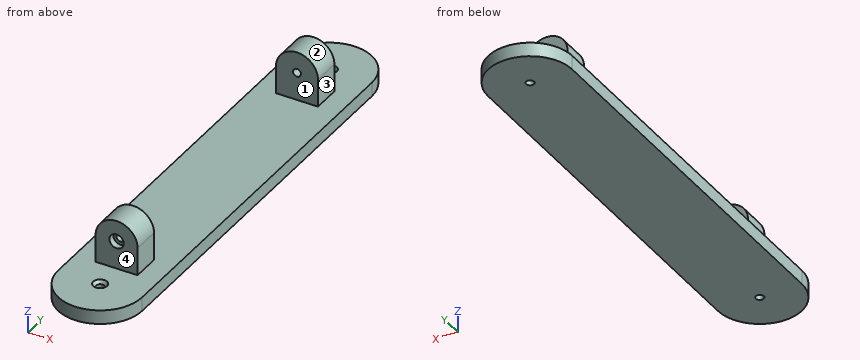
from build123d import *

# Parameters (mm, degrees)
BOSS_EXTRUDE1_DEPTH                             = 6.35
CSK_FOR_M3_FLAT_HEAD_MACHINE_SCREW1_D           = 3.6
CSK_FOR_M3_FLAT_HEAD_MACHINE_SCREW1_CSINK_D     = 6.3
CSK_FOR_M3_FLAT_HEAD_MACHINE_SCREW1_CSINK_ANGLE = 90
SKETCH3_W                                       = 19.05
SKETCH3_H                                       = 12.7
BOSS_EXTRUDE2_DEPTH                             = 12.7
BOSS_EXTRUDE5_DEPTH                             = 12.7
CBORE_FOR_M3_SHCS1_D                            = 3.6
CBORE_FOR_M3_SHCS1_CBORE_D                      = 6.5
CBORE_FOR_M3_SHCS1_CBORE_DEPTH                  = 3


with BuildPart() as part:
    # Sketch1 → Boss-Extrude1 (new body)
    with BuildSketch(Plane.XY):
        with BuildLine():
            Line((0, 0), (38.1, 0))
            Line((38.1, 0), (38.1, 88.9))
            ThreePointArc((38.1, 88.9), (19.05, 107.95), (0, 88.9))
            Line((0, 88.9), (0, 0))
        make_face()
    boss_extrude1 = extrude(amount=BOSS_EXTRUDE1_DEPTH)

    # CSK for M3 Flat Head Machine Screw1 (through all)
    with Locations(Plane(origin=(19.05, 88.9, 6.35), x_dir=(1, 0, 0), z_dir=(0, 0, 1))):
        with Locations((0, 0)):
            csk_for_m3_flat_head_machine_screw1 = CounterSinkHole(CSK_FOR_M3_FLAT_HEAD_MACHINE_SCREW1_D / 2, CSK_FOR_M3_FLAT_HEAD_MACHINE_SCREW1_CSINK_D / 2, counter_sink_angle=CSK_FOR_M3_FLAT_HEAD_MACHINE_SCREW1_CSINK_ANGLE)

    # Sketch3 → Boss-Extrude2 (add)
    with BuildSketch(Plane.XY.offset(6.35)):
        with Locations((19.05, 69.85)):
            Rectangle(SKETCH3_W, SKETCH3_H)
    boss_extrude2 = extrude(amount=BOSS_EXTRUDE2_DEPTH)

    # Sketch6 → Boss-Extrude5 (add)
    with BuildSketch(Plane(origin=(0, 76.2, 0), x_dir=(1, 0, 0), z_dir=(0, 1, 0))):
        with BuildLine():
            Line((9.525, -19.05), (28.575, -19.05))
            ThreePointArc((28.575, -19.05), (19.05, -28.575), (9.525, -19.05))
        make_face()
    boss_extrude5 = extrude(amount=-BOSS_EXTRUDE5_DEPTH)

    # CBORE for M3 SHCS1 (through all)
    with Locations(Plane(origin=(0, 76.2, 0), x_dir=(1, 0, 0), z_dir=(0, 1, 0))):
        with Locations((19.05, -19.05)):
            cbore_for_m3_shcs1 = CounterBoreHole(CBORE_FOR_M3_SHCS1_D / 2, CBORE_FOR_M3_SHCS1_CBORE_D / 2, CBORE_FOR_M3_SHCS1_CBORE_DEPTH)

    # Mirror1: Boss-Extrude1, CSK for M3 Flat Head Machine Screw1, Boss-Extrude2, Boss-Extrude5, CBORE for M3 SHCS1 across plane
    add(boss_extrude1.mirror(Plane.ZX))
    add(csk_for_m3_flat_head_machine_screw1.mirror(Plane.ZX), mode=Mode.SUBTRACT)
    add(boss_extrude2.mirror(Plane.ZX))
    add(boss_extrude5.mirror(Plane.ZX))
    add(cbore_for_m3_shcs1.mirror(Plane.ZX), mode=Mode.SUBTRACT)


solid = part.part
Work out the finished part from the listing and answer in its coordinate system (mm). Face numbers are marked on the shaded views. A direction names the side the tool comes from. Coordinates: 2 decimals unless noted, no trailing zeros. Write each loop counter-clockwise with the first axis right and the second up, starting at its lowest first coordinate (ties: lowest second). Pieces come first, ordered by that corner, then holes.
1. The part is cut by section C-C, the plane x = 13. Write down the section's boundary in (y, z), and give its area (3 significant figures).
Results list:
outline: (-106.96, 0) - (106.96, 0) - (106.96, 6.35) - (76.2, 6.35) - (76.2, 26.41) - (63.5, 26.41) - (63.5, 6.35) - (-63.5, 6.35) - (-63.5, 26.41) - (-76.2, 26.41) - (-76.2, 6.35) - (-106.96, 6.35) - close
area: 1,870 mm2
2. The part is cut by section D-D, the plane z = 25.75. Write down the section's boundary in (x, y).
Results list:
outline: (12.28, -76.2) - (25.82, -76.2) - (25.82, -63.5) - (12.28, -63.5) - close; (12.28, 63.5) - (25.82, 63.5) - (25.82, 76.2) - (12.28, 76.2) - close
3. The part is cut by section B-B, the plane z = 12.5. Write down the section's boundary in (x, y) (3 decimals), and give its area (3 significant figures).
Results list:
outline: (9.525, -76.2) - (28.575, -76.2) - (28.575, -63.5) - (9.525, -63.5) - close; (9.525, 63.5) - (28.575, 63.5) - (28.575, 76.2) - (9.525, 76.2) - close
area: 484 mm2
4. For the marked faces 1, 2, 3 and 4, determine the directions among +Z, -Z, +X, -X, +Y, -Y from which every point of the face is accessible in a straight line to the end or side of a thin tool.
Results list:
face 1: +Z, +X, -X
face 2: +Z, +Y, -Y
face 3: +Z, +X, +Y, -Y
face 4: +Z, +X, -X, -Y
5. The part is cut by section A-A, the plane y = 70. Write down the section's boundary in (x, z) (3 decimals), and give its area (3 significant figures).
Results list:
outline: (0, 0) - (38.1, 0) - (38.1, 6.35) - (28.575, 6.35) - (28.575, 19.05) arc R9.525 ccw to (9.525, 19.05) - (9.525, 6.35) - (0, 6.35) - close; hole circle Ø3.6 at (19.05, 19.05)
area: 616 mm2
6. Flat-ended cylindrical pins translate along their axes: pin 1 (8.5 mm diameter, centred on x = 19.05, z = 19.05, fed in from +Y); pin 2 (2 mm diameter, centred on x = 30, z = 15.5, fed in from -Y); pin 3 (3 mm diameter, centred on x = 19, z = 19.5, fed in from +Y); pin 4 (12 mm diameter, centred on y = 76, z = 16, fed in from -X) (3 decimals). Find the tip coordinate at first contact, or state that the pin passes through.
Results list:
pin 1: stops at y = 76.2
pin 2: passes through
pin 3: stops at y = 73.2
pin 4: stops at x = 9.525
7. Consider line 1 along Y through (x, z) = (19.05, 2.6); line 2 along Y through (x, z) = (20.5, 7.5); line 3 along X through (y, z) = (-69.5, 19.05) (3 decimals). Determine where each line is inside the solid, lowest interval first.
Results list:
line 1: y = -107.95 to -90.7, -87.1 to 87.1, 90.7 to 107.95
line 2: y = -76.2 to -63.5, 63.5 to 76.2
line 3: x = 9.525 to 17.25, 20.85 to 28.575
